Autodesk Inventor part; units mm, degrees
ref_plane "Płaszczyzna konstrukcyjna1" through (0, 0, 0) normal (0, 0, 1) x (1, 0, 0)
ref_plane "YZ Plane" through (0, 0, 0) normal (1, 0, 0) x (0, 1, 0)
ref_plane "XZ Plane" through (0, 0, 0) normal (0, 1, 0) x (-1, 0, 0)
ref_plane "Płaszczyzna konstrukcyjna1" through (0, 0, 0) normal (0, 0, 1) x (1, 0, 0)
sketch "Szkic1" plane through (0, 0, 0) normal (0, 0, 1) x (1, 0, 0)
  circle A0 centre (-13, -22.5167) radius 2.5
  circle A1 centre (-13, -22.5167) radius 2.5
  point P0 (0, 0)
extrude "Wyciągnięcie proste1" add sketch "Szkic1" against normal blind 11
sketch "Szkic2" plane through (-13, -22.5167, -11) normal (0, 0, -1) x (-1, 0, 0)
  circle A0 centre (0, 0) radius 2.5
  circle A1 centre (0, 0) radius 3.5
  point P0 (-13, 22.5167)
  dimension "d2" = 7
extrude "Wyciągnięcie proste2" add sketch "Szkic2" along normal blind 1.5 contours A0 | A1
sketch "Szkic3" plane through (-13, -22.5167, 0) normal (0, 0, 1) x (1, 0, 0)
  circle A0 centre (0, 0) radius 3.5
  point P0 (13, 22.5167)
  dimension "d5" = 7
extrude "Wyciągnięcie proste3" add sketch "Szkic3" along normal blind 1.5
properties part number "Nit tarczy długi" material "Stal, węglowa"
Can you work these out from the model? Positions are in its coordinate system, mm. A direction names the side the tool comes from. Give positions to 0.01 mm unless a question says otherwise; leave off trailing zeros. Order: outer loops, then holes, each group sorted by start corner. A loop starts at its lowest first (then second) coordinate and runs counter-clockwise, first axis right, second up. Notation, with made-up numbers: (65.25, 77) - (106.25, 77) arc R20 ccw to (106.25, 97) - close; hole circle Ø10 at (26, 54.25). An arc over 180 degrees is marked (long way). Use a Markdown table: item, result. Add a question column.
Q1. If we section it at D-D on y = -19.5: Write out the boundary of the cut face in (x, z).
Q2. Please list where these lines run through material, in increasing order: line 1 along Z through (x, y) = (-11, -20.75); line 2 along Y through (x, z) = (-13, -4.5); line 3 along Y through (x, z) = (-10.75, -5.5).
Q3. If we section it at B-B on y = -25.25: Write out the boundary of the cut face in (x, z).
Q4. On a 3-axis mill with a long thin cutter (end or side, diameter ignored), from which of +Z, -Z, +X, -X, +Y, -Y can I reach the whole of each face in a straight line? I mean faces 4 (the flat face through (-13, -22, -12.5)), 5 (the flat face through (-14, -20, 0)). Say none if no direction works.
Q5. If we section it at C-C on y = -22: Write out the boundary of the cut face in (x, z).
Q6. If we section it at A-A on x = -13: Write out the boundary of the cut face in (y, z), plus the area to 3 significant figures.
Q7. If we mould it in two halves opening along Z, with no side actions, what happens to faces 1 (the flat face through (-12, -20, -11)), 2 (the cylindrical face through (-13.456, -25.987, 0.74)), 3 (the flat face through (-13, -22, 1.5))? For each: released by +Z, released by -Z, zero draft, split by the parting line, or undercut.
Q8. I'm going to push flat-ended pins straight in: pin 1 (1.5 mm diameter, centred on y = -23.5, z = 0, fed in from -X); pin 2 (1 mm diameter, centred on y = -22.5, z = -1, fed in from -X); pin 3 (1 mm diameter, centred on x = -10.5, z = -10, fed in from +Y). Where does each tip first touch, or does it pass through?
Answers follow:
| question | item | result |
|---|---|---|
| 1 | outline | (-14.77, -12.5) - (-11.23, -12.5) - (-11.23, -11) - (-14.77, -11) - close; (-14.77, 0) - (-11.23, 0) - (-11.23, 1.5) - (-14.77, 1.5) - close |
| 2 | line 1 | z = -12.5 to -11, 0 to 1.5 |
| 2 | line 2 | y = -25.02 to -20.02 |
| 2 | line 3 | y = -23.61 to -21.43 |
| 3 | outline | (-15.19, -12.5) - (-10.81, -12.5) - (-10.81, -11) - (-15.19, -11) - close; (-15.19, 0) - (-10.81, 0) - (-10.81, 1.5) - (-15.19, 1.5) - close |
| 4 | face 4 | -Z, +X, -X, +Y, -Y |
| 4 | face 5 | none |
| 5 | outline | (-16.46, -12.5) - (-9.54, -12.5) - (-9.54, -11) - (-10.55, -11) - (-10.55, 0) - (-9.54, 0) - (-9.54, 1.5) - (-16.46, 1.5) - (-16.46, 0) - (-15.45, 0) - (-15.45, -11) - (-16.46, -11) - close |
| 6 | outline | (-26.02, -12.5) - (-19.02, -12.5) - (-19.02, -11) - (-20.02, -11) - (-20.02, 0) - (-19.02, 0) - (-19.02, 1.5) - (-26.02, 1.5) - (-26.02, 0) - (-25.02, 0) - (-25.02, -11) - (-26.02, -11) - close |
| 6 | area | 76.0 mm^2 |
| 7 | face 1 | undercut |
| 7 | face 2 | zero draft |
| 7 | face 3 | released by +Z |
| 8 | pin 1 | stops at x = -16.49 |
| 8 | pin 2 | stops at x = -15.5 |
| 8 | pin 3 | stops at y = -21.02 |
